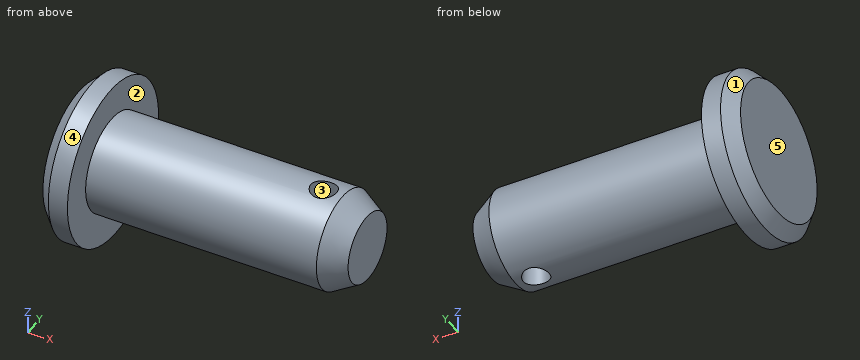
Autodesk Inventor part; units mm, degrees
ref_plane "Work Plane1" through (16, 0, 6) normal (0, 0, 1) x (1, 0, 0)
ref_plane "YZ Plane" through (0, 0, 0) normal (1, 0, 0) x (0, 1, 0)
ref_plane "XZ Plane" through (0, 0, 0) normal (0, 1, 0) x (-1, 0, 0)
sketch "Skizze1" plane through (0, 0, 0) normal (0, 0, 1) x (1, 0, 0)
  line L0 (-4, 0) -> (-4, 10)
  line L1 (-4, 10) -> (0, 10)
  line L2 (0, 10) -> (0, 6)
  line L3 (0, 6) -> (32, 6)
  line L4 (32, 6) -> (32, 0)
  line L5 (-4, 0) -> (32, 0)
  line L6 (-4, 0) -> (17, 0)
  line L7 (0, -0.98) -> (0, 3.08)
  circle A0 centre (26.5, 0) radius 1.6
  dimension "d0" = 12
  dimension "d1" = 20
  dimension "d2" = 4
  dimension "d3" = 32
  dimension "d5" = 5.5
  dimension "d6" = 3.2
revolve "Körper" add sketch "Skizze1" angle 360 about axis through (-4, 0, 0) along (1, 0, 0) picked at (26.9216, 0.9202) contours L0 L1 L2 L3 L4 L5 A0 | A0 L5
extrude "Bohrung" cut sketch "Skizze1" along normal through all both and the other way through all contours A0 L5 | L5 A0
chamfer "Fase1" distance 1.6 angle 45 1 edges at (-4, -10, 0) measured on face at (-2.6667, 9.9676, -0.8047)
chamfer "Fase2" distance 3 angle 30 1 edges at (32, -6, 0) measured on face at (19.4513, 2.8362, 5.2873)
ref_plane "Work Plane1" through (16, 0, 6) normal (0, 0, 1) x (1, 0, 0)
equation "\"d0\" = NND"
equation "\"d1\" = KOD"
equation "\"d2\" = KOH"
equation "\"d3\" = NLG"
equation "\"d5\" = DIST"
equation "\"d6\" = BOR"
equation "\"d7\" = NND"
equation "\"d9\" = PHH2"
equation "\"d10\" = FAWI2"
equation "\"d16\" = PHH2"
equation "\"d11\" = PHH1"
equation "\"d12\" = FAWI1"
equation "\"d17\" = PHH1"
equation "\"PHH1\" = 3"
equation "\"PHH2\" = 1.6"
equation "\"KOD\" = 20"
equation "\"KOH\" = 4"
equation "\"NND\" = 12"
equation "\"FAWI1\" = 30deg"
equation "\"FAWI2\" = 45deg"
equation "\"DIST\" = 5.5"
equation "\"BOR\" = 3.2"
equation "\"NLG\" = 32"
properties part number "IS 6863 - B12 x 32" material "Stahl, weich"
The listing builds one solid part. Answer for the finished solid, in the listing's coordinates (mm). Face numbers are marked on the shaded views. A direction names the side the tool comes from. Give positions to 0.01 mm unless a question says otherwise; leave off trailing zeros. Order: outer loops, then holes, each group sorted by start corner. A loop starts at its lowest first (then second) coordinate and runs counter-clockwise, first axis right, second up.
Item 1: The part is cut by section B-B, the plane z = 0. Give the vertices of the cut face in (x, y).
From the geometry:
outline: (-4, -8.4) - (-2.4, -10) - (0, -10) - (0, -6) - (29, -6) - (32, -4.27) - (32, 4.27) - (29, 6) - (0, 6) - (0, 10) - (-2.4, 10) - (-4, 8.4) - close; hole circle Ø3.2 at (26.5, 0)
Item 2: The part is cut by section A-A, the plane y = 0. Give the vertices of the cut face in (x, z), and give its area (3 significant figures).
From the geometry:
outline: (-4, -8.4) - (-2.4, -10) - (0, -10) - (0, -6) - (24.9, -6) - (24.9, 6) - (0, 6) - (0, 10) - (-2.4, 10) - (-4, 8.4) - close; (28.1, -6) - (29, -6) - (32, -4.27) - (32, 4.27) - (29, 6) - (28.1, 6) - close
area: 418 mm2
Item 3: For a pull along Y with two mould halves and no side action, classify the marked faces 3, 4 and 5 as pulls with the +Y half, pulls with the -Y half, needs draft (parallel to the pull), parting line crosses it, or undercut.
From the geometry:
face 3: undercut
face 4: parting line crosses it
face 5: needs draft
Item 4: Find the intervals of material crossed by probe 1 along X at (y, z) = (0, 0.75); probe 2 along Y at (x, z) = (26.5, -0.25); probe 3 along X at (y, z) = (-7, -3.25), in increasing order.
From the geometry:
probe 1: x = -4 to 24.9, 28.1 to 32
probe 2: y = -5.99 to -1.6, 1.6 to 5.99
probe 3: x = -4 to 0
Item 5: Given pin 1 Ø8 at (x, y) = (3, -6) entering from -Z; pin 2 Ø4 at (x, y) = (26.5, 0) entering from -Z; pin 3 Ø4 at (y, z) = (-1.5, -6.5) entering from +X; pin 4 Ø2 at (x, y) = (3, -7.5) entering from +Z, each flat-ended and moving along its own axis, determine where each tip first touches the part or whether it passes through.
From the geometry:
pin 1: stops at z = -9.42
pin 2: stops at z = -6
pin 3: stops at x = 31.3
pin 4: passes through
Item 6: The part is cut by section C-C, the plane x = 24. Give the vertices of the cut face in (y, z), and give its area (3 significant figures).
From the geometry:
outline: circle Ø12 at (0, 0)
area: 113 mm2
Item 7: Which of the six approach directions +Z, -Z, +X, -X, +Y, -Y give full straight-line access (tool end or side, diameter ignored) to the marked faces 1 and 2?
From the geometry:
face 1: -X
face 2: +X
